Geometry check sheet. Reference: the model listing, model coordinates, mm. Face numbers are marked on the shaded views. Give positions to 0.01 mm unless a question says otherwise; leave off trailing zeros. Write each loop counter-clockwise with the first axis right and the second up, starting at its lowest first coordinate (ties: lowest second). Pieces come first, ordered by that corner, then holes. Notation, with made-up numbers: (33, -21) - (84, -21) arc R7 ccw to (84, -15) - close; hole circle Ø10 at (64, 25.5). An arc over 180 degrees is marked (long way). One line per question, with ' | ' between items. Start each with the question number.
Q1. Section check D-D on z = 86.5. Record the boundary of the cut face in (x, y), and give its area (3 significant figures).
Q2. Release check for a two-part mould opening along Y. For the marked faces 1, 2 and 3 record: +Y half, -Y half, draft (parallel to the pull), parting line (faces both ways), or undercut.
Q3. Section check A-A on z = 15.5. Record the boundary of the cut face in (x, y) (3 decimals).
Q4. Thickness scan on L1, parallel to Z at x = -104, y = 18; L2, parallel to Z at x = -59, y = -10.5; L3, parallel to X at y = -20, z = 22. Record the ranges inside material, lowest first. Write a range as [from, to].
Q5. Gauge pin test, flat ends, axial feed: P1, Ø5, axis at x = -69, y = 26.5, coming from the -Z side; P2, Ø10, axis at x = -91.5, y = 18.5, coming from the +Z side. Record the tip position at first contact, or that the pin passes through.
Q6. Section check C-C on y = -18.5. Record the boundary of the cut face in (x, z), and give its area (3 significant figures).
Q7. Section check B-B on x = -118. Record the boundary of the cut face in (y, z), and give its area (3 significant figures).
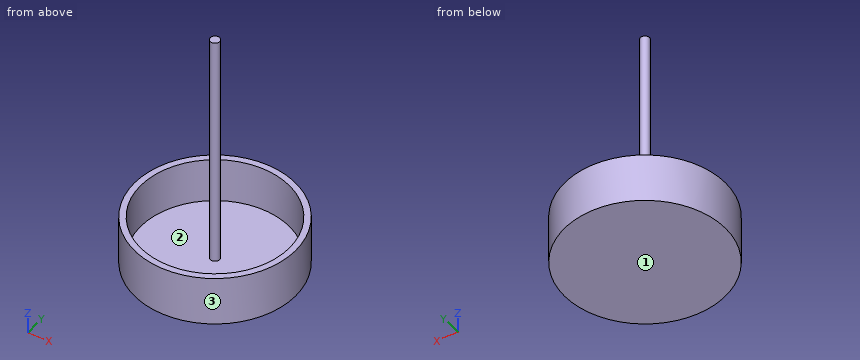
```python
from build123d import *

# Parameters (mm, degrees)
F0_R     = 38.1
F0_R_2   = 2.413
F1_DEPTH = 2.54
F0_R_3   = 41.275
F2_DEPTH = 25.4
F3_R     = 2.413
F4_DEPTH = 124.46


with BuildPart() as f1:
    # F0 (on Top) → F1 (new body)
    with BuildSketch(Plane.XY):
        with Locations((-94.074033, 5.041726)):
            Circle(F0_R)
        with Locations((-94.074033, 5.041726)):
            Circle(F0_R_2, mode=Mode.SUBTRACT)
    extrude(amount=F1_DEPTH)

    # F0 (on Top) → F2 (join)
    with BuildSketch(Plane.XY):
        with Locations((-94.074033, 5.041726)):
            Circle(F0_R_3)
        with Locations((-94.074033, 5.041726)):
            Circle(F0_R, mode=Mode.SUBTRACT)
    extrude(amount=F2_DEPTH)

    # F3 (on face) → F4 (join)
    with BuildSketch(Plane.XY):
        with Locations((-94.074033, 5.041726)):
            Circle(F3_R)
    extrude(amount=F4_DEPTH)


solid = f1.part
```
Working result:
1) outline: circle Ø4.83 at (-94.07, 5.04) | area: 18.3 mm2
2) face 1: draft | face 2: undercut | face 3: parting line
3) outline: circle Ø82.55 at (-94.074, 5.042); circle Ø4.826 at (-94.074, 5.042); hole circle Ø76.2 at (-94.074, 5.042)
4) L1: z = [0, 2.54] | L2: z = [0, 25.4] | L3: x = [-126.88, -122.79], [-65.36, -61.26]
5) P1: stops at z = 0 | P2: stops at z = 2.54
6) outline: (-127.98, 0) - (-60.17, 0) - (-60.17, 25.4) - (-64.12, 25.4) - (-64.12, 2.54) - (-124.03, 2.54) - (-124.03, 25.4) - (-127.98, 25.4) - close | area: 353 mm2
7) outline: (-28.59, 0) - (38.67, 0) - (38.67, 25.4) - (34.69, 25.4) - (34.69, 2.54) - (-24.61, 2.54) - (-24.61, 25.4) - (-28.59, 25.4) - close | area: 353 mm2
